Design review of the part built by this model. Coordinates are the model's own, in mm. A direction names the side the tool comes from. Round coordinates to 2 decimals unless told otherwise and drop trailing zeros. Order: outer loops, then holes, each group sorted by start corner. A loop starts at its lowest first (then second) coordinate and runs counter-clockwise, first axis right, second up. Notation, with made-up numbers: (89, 14) - (121, 14) arc R22 cw to (121, 48) - close; hole circle Ø10 at (64.5, 23.25). An arc over 180 degrees is marked (long way). Use CSV: the item, a comma, the result in double quotes.
from build123d import *

# Parameters (mm, degrees)
SKETCH1_R           = 30.3
BOSS_EXTRUDE1_DEPTH = 106
CUT_EXTRUDE1_REACH  = 108
SKETCH2_W           = 5
SKETCH2_H           = 60.6
SHELL1_T            = -1.8
CUT_EXTRUDE2_REACH  = 3.8
SKETCH3_R           = 1.75
SKETCH3_R_2         = 7.5
SKETCH4_W           = 7
SKETCH4_H           = 8
SKETCH4_R           = 1.75
BOSS_EXTRUDE2_DEPTH = 15


with BuildPart() as part:
    # Sketch1 → Boss-Extrude1 (new body)
    with BuildSketch(Plane(origin=(0, 0, 0), x_dir=(1, 0, 0), z_dir=(0, 1, 0))):
        Circle(SKETCH1_R)
    extrude(amount=BOSS_EXTRUDE1_DEPTH)

    # Sketch2 → Cut-Extrude1 (cut, up to next)
    with BuildSketch(Plane(origin=(0, 106, 0), x_dir=(1, 0, 0), z_dir=(0, 1, 0)), mode=Mode.PRIVATE) as cut_extrude1_sk1:
        with Locations((28.5, 0)):
            Rectangle(SKETCH2_W, SKETCH2_H)
    cut_extrude1_tool1 = extrude(cut_extrude1_sk1.sketch, amount=-CUT_EXTRUDE1_REACH, mode=Mode.PRIVATE) & part.part
    add(cut_extrude1_tool1.solids().sort_by_distance((28.5, 106, 0))[0], mode=Mode.SUBTRACT)
    # Sketch2 → Cut-Extrude1 (cut, up to next)
    with BuildSketch(Plane(origin=(0, 106, 0), x_dir=(1, 0, 0), z_dir=(0, 1, 0)), mode=Mode.PRIVATE) as cut_extrude1_sk2:
        with Locations((-28.5, 0)):
            Rectangle(SKETCH2_W, SKETCH2_H)
    cut_extrude1_tool2 = extrude(cut_extrude1_sk2.sketch, amount=-CUT_EXTRUDE1_REACH, mode=Mode.PRIVATE) & part.part
    add(cut_extrude1_tool2.solids().sort_by_distance((-28.5, 106, 0))[0], mode=Mode.SUBTRACT)

    # Shell1
    shell1_openings = [part.faces().sort_by_distance(p)[0] for p in [
        (0, 106, 0),
    ]]
    offset(amount=SHELL1_T, openings=shell1_openings, kind=Kind.INTERSECTION)

    # Sketch3 → Cut-Extrude2 (cut, up to next)
    with BuildSketch(Plane(origin=(0, 1.8, 0), x_dir=(1, 0, 0), z_dir=(0, 1, 0)), mode=Mode.PRIVATE) as cut_extrude2_sk1:
        with Locations((0, 23.5)):
            Circle(SKETCH3_R)
    cut_extrude2_tool1 = extrude(cut_extrude2_sk1.sketch, amount=-CUT_EXTRUDE2_REACH, mode=Mode.PRIVATE) & part.part
    add(cut_extrude2_tool1.solids().sort_by_distance((0, 1.8, -23.5))[0], mode=Mode.SUBTRACT)
    # Sketch3 → Cut-Extrude2 (cut, up to next)
    with BuildSketch(Plane(origin=(0, 1.8, 0), x_dir=(1, 0, 0), z_dir=(0, 1, 0)), mode=Mode.PRIVATE) as cut_extrude2_sk2:
        with Locations((0, -23.5)):
            Circle(SKETCH3_R)
    cut_extrude2_tool2 = extrude(cut_extrude2_sk2.sketch, amount=-CUT_EXTRUDE2_REACH, mode=Mode.PRIVATE) & part.part
    add(cut_extrude2_tool2.solids().sort_by_distance((0, 1.8, 23.5))[0], mode=Mode.SUBTRACT)
    # Sketch3 → Cut-Extrude2 (cut, up to next)
    with BuildSketch(Plane(origin=(0, 1.8, 0), x_dir=(1, 0, 0), z_dir=(0, 1, 0)), mode=Mode.PRIVATE) as cut_extrude2_sk3:
        Circle(SKETCH3_R_2)
    cut_extrude2_tool3 = extrude(cut_extrude2_sk3.sketch, amount=-CUT_EXTRUDE2_REACH, mode=Mode.PRIVATE) & part.part
    add(cut_extrude2_tool3.solids().sort_by_distance((0, 1.8, 0))[0], mode=Mode.SUBTRACT)

    # Sketch4 → Boss-Extrude2 (add)
    with BuildSketch(Plane(origin=(0, 1.8, 0), x_dir=(1, 0, 0), z_dir=(0, 1, 0))):
        with Locations((0, 24.5)):
            Rectangle(SKETCH4_W, SKETCH4_H)
        with Locations((0, 23.5)):
            Circle(SKETCH4_R, mode=Mode.SUBTRACT)
        with Locations((0, -24.5)):
            Rectangle(SKETCH4_W, SKETCH4_H)
        with Locations((0, -23.5)):
            Circle(SKETCH4_R, mode=Mode.SUBTRACT)
    extrude(amount=BOSS_EXTRUDE2_DEPTH)


solid = part.part
1) Insertion check: pin 1 Ø3 at (x, z) = (0, -23.5) entering from -Y; pin 2 Ø6 at (y, z) = (12.5, -23) entering from +X; pin 3 Ø8 at (x, y) = (-8.5, 80) entering from +Z; pin 4 Ø7.5 at (x, y) = (1.5, 7) entering from -Z. Each pin has a flat end and moves straight along its axis. Give the tip position at first contact, or say it passes through.
Data:
pin 1,"passes through"
pin 2,"stops at x = 22.76"
pin 3,"stops at z = 29.96"
pin 4,"stops at z = -30.3"
2) We need section C-C (y = 83.5). Give the boundary of the cut face in (x, z), then the cut area to 3 significant figures.
Data:
outline,"(-26, -15.56) arc R30.3 ccw to (26, -15.56) - (26, 15.56) arc R30.3 ccw to (-26, 15.56) - close; hole (-24.2, -15.05) arc R28.5 ccw to (24.2, -15.05) - (24.2, 15.05) arc R28.5 ccw to (-24.2, 15.05) - close"
area,"327 mm2"
3) To check wall thickness, follow L1, parallel to Z at x = 0, y = 7.25; L2, parallel to Z at x = 0, y = 1.3; L3, parallel to X at y = 37, z = -15. State the ranges of each line that lie inside material, in increasing order. Write a range as from..to.
Data:
L1,"z = -30.3..-25.25, -21.75..-20.5, 20.5..21.75, 25.25..30.3"
L2,"z = -30.3..-25.25, -21.75..-7.5, 7.5..21.75, 25.25..30.3"
L3,"x = -26..-24.2, 24.2..26"
4) We need section B-B (z = 5.5). Give the boundary of the cut face in (x, y), then the cut area to 3 significant figures.
Data:
outline,"(-26, 0) - (-5.1, 0) - (-5.1, 1.8) - (-24.2, 1.8) - (-24.2, 106) - (-26, 106) - close; (5.1, 0) - (26, 0) - (26, 106) - (24.2, 106) - (24.2, 1.8) - (5.1, 1.8) - close"
area,"450 mm2"
5) For faces 1 (the face through (-0.05, 16.8, -25.44)), 2 (the face through (-0.438, 52.258, 30.297)), list the 3-axis set-ups (+Z, -Z, +X, -X, +Y, -Y) from which the entire face can be reached by the end or side of a thin tool; tool diameter is ignored.
Data:
face 1,"+Y"
face 2,"+Z, +Y, -Y"
6) The part is to be moulded in two halves that separate along Z. For faces 3 (the face through (5, 0, 6)), 4 (the face through (3.5, 9, -24)), 5 (the face through (0.438, 52.258, -30.297)), say which applies: +Z half, -Z half, draft (parallel to the pull), parting line (faces both ways), or undercut.
Data:
face 3,"draft"
face 4,"undercut"
face 5,"-Z half"
7) We need section D-D (z = -9). Give the boundary of the cut face in (x, y), then the cut area to 3 significant figures.
Data:
outline,"(-26, 0) - (26, 0) - (26, 106) - (24.2, 106) - (24.2, 1.8) - (-24.2, 1.8) - (-24.2, 106) - (-26, 106) - close"
area,"469 mm2"
8) We need section A-A (x = 0). Give the boundary of the cut face in (y, z), then the cut area to 3 significant figures.
Data:
outline,"(0, -30.3) - (106, -30.3) - (106, -28.5) - (16.8, -28.5) - (16.8, -25.25) - (0, -25.25) - close; (0, -21.75) - (16.8, -21.75) - (16.8, -20.5) - (1.8, -20.5) - (1.8, -7.5) - (0, -7.5) - close; (0, 7.5) - (1.8, 7.5) - (1.8, 20.5) - (16.8, 20.5) - (16.8, 21.75) - (0, 21.75) - close; (0, 25.25) - (16.8, 25.25) - (16.8, 28.5) - (106, 28.5) - (106, 30.3) - (0, 30.3) - close"
area,"580 mm2"
